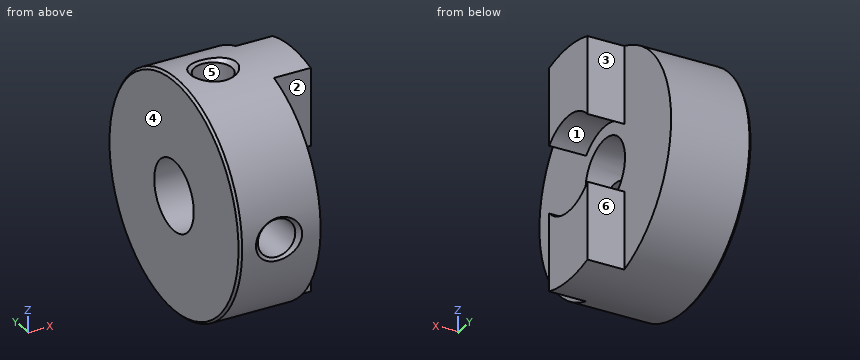
from build123d import *

# Parameters (mm, degrees)
SKETCH2_W          = 3.2
SKETCH2_H          = 4.1
SKETCH3_W          = 22
SKETCH3_H          = 21
SKETCH3_W_2        = 20
SKETCH3_H_2        = 5.8
CUT_EXTRUDE1_DEPTH = 3.2


with BuildPart() as part:
    # Sketch1 → Revolve1 (revolve)
    with BuildSketch(Plane.XY):
        Polygon((0, 9.8), (0, 3), (10.2, 3), (10.2, 10), (0.2, 10), align=None)
    revolve(axis=Axis((10.2, 0, 0), (-1, 0, 0)))

    # Sketch2 → Cut-Revolve1 (revolve, cut)
    with BuildSketch(Plane.XY):
        with Locations((8.6, 2.05)):
            Rectangle(SKETCH2_W, SKETCH2_H)
    revolve(axis=Axis((10.2, 0, 0), (-1, 0, 0)), mode=Mode.SUBTRACT)

    # Sketch3 → Cut-Extrude1 (cut)
    with BuildSketch(Plane(origin=(10.2, 0, 0), x_dir=(0, 0, -1), z_dir=(1, 0, 0))):
        Rectangle(SKETCH3_W, SKETCH3_H)
        Rectangle(SKETCH3_W_2, SKETCH3_H_2, mode=Mode.SUBTRACT)
    extrude(amount=-CUT_EXTRUDE1_DEPTH, mode=Mode.SUBTRACT)

    # Sketch4 → Cut-Revolve2 (revolve, cut)
    with BuildSketch(Plane(origin=(3.4, 0, 0), x_dir=(0, 0, -1), z_dir=(1, 0, 0))):
        Polygon((-10, 0), (-10, 2), (-9.621, 1.621), (0, 1.621), (0, 0), align=None)
    revolve(axis=Axis((3.4, 0, 0), (0, 0, 1)), mode=Mode.SUBTRACT)

    # Sketch5 → Cut-Revolve3 (revolve, cut)
    with BuildSketch(Plane(origin=(3.4, 0, 0), x_dir=(0, 0, -1), z_dir=(1, 0, 0))):
        Polygon((0, -10), (-2, -10), (-1.621, -9.621), (-1.621, 0), (0, 0), align=None)
    revolve(axis=Axis((3.4, 0, 0), (0, -1, 0)), mode=Mode.SUBTRACT)


solid = part.part
Source: CAD feature listing. Evaluate the final solid. Frame: model axes, mm. Face numbers are marked on the shaded views. A direction names the side the tool comes from. Coordinates: 2 decimals unless noted, no trailing zeros. Write each loop counter-clockwise with the first axis right and the second up, starting at its lowest first coordinate (ties: lowest second). Pieces come first, ordered by that corner, then holes. Notation, with made-up numbers: M 48.25,64 L 99.25,64 A11 cw 99.25,78 Z; hole C -15,87 d4. An arc over 180 degrees is marked long. Use a Markdown table: item, result.
1) Ray query, L1, parallel to Y at x = 2, z = 0; L2, parallel to X at y = 6.25, z = -1.25; L3, parallel to Z at x = 1.75, y = 2.75. Return the intervals inside material, ascending.
Conclusion:
| item | result |
|---|---|
| L1 | y = 3 to 10 |
| L2 | x = 0 to 7 |
| L3 | z = -9.61 to -1.2, 1.2 to 9.61 |
2) Mould query, pull axis Y, two halves, no side actions, for the marked faces 4, 5 and 6. Classes: pulls with the +Y half, pulls with the -Y half, needs draft (parallel to the pull), parting line crosses it, or undercut.
Conclusion:
| item | result |
|---|---|
| face 4 | needs draft |
| face 5 | undercut |
| face 6 | pulls with the +Y half |
3) First-contact query: pin 1 Ø10 at (y, z) = (5, 6) entering from -X; pin 2 Ø6 at (x, z) = (2.5, 3) entering from -Y; pin 3 Ø1.6 at (x, z) = (8.5, -5.5) entering from +Y; pin 4 Ø6 at (x, y) = (6, -4) entering from -Z. Flat tips, straight axial feed; report the tip coordinate or a pass-through.
Conclusion:
| item | result |
|---|---|
| pin 1 | stops at x = 0 |
| pin 2 | stops at y = -10 |
| pin 3 | stops at y = 2.9 |
| pin 4 | stops at z = -9.95 |
4) Section C-C, the plane x = 8.25. Output: boundary loops of the cut face in (y, z), then the cut area to 3 significant figures.
Conclusion:
| item | result |
|---|---|
| outline | M -2.9,-9.57 A10 ccw 2.9,-9.57 L 2.9,-2.9 A4.1 cw -2.9,-2.9 Z; M -2.9,2.9 A4.1 cw 2.9,2.9 L 2.9,9.57 A10 ccw -2.9,9.57 Z |
| area | 71.1 mm^2 |
5) Section A-A, the plane y = 0. Output: boundary loops of the cut face in (x, z).
Conclusion:
| item | result |
|---|---|
| outline | M 0,-9.8 L 0.2,-10 L 10.2,-10 L 10.2,-4.1 L 7,-4.1 L 7,-3 L 0,-3 Z; M 0,3 L 1.78,3 L 1.78,9.62 L 1.4,10 L 0.2,10 L 0,9.8 Z; M 5.02,3 L 7,3 L 7,4.1 L 10.2,4.1 L 10.2,10 L 5.4,10 L 5.02,9.62 Z |
6) Section B-B, the plane z = 0. Output: boundary loops of the cut face in (x, y), then the cut area to 3 significant figures.
Conclusion:
| item | result |
|---|---|
| outline | M 0,-9.8 L 0.2,-10 L 1.4,-10 L 1.78,-9.62 L 1.78,-3 L 0,-3 Z; M 0,3 L 7,3 L 7,10 L 0.2,10 L 0,9.8 Z; M 5.02,-9.62 L 5.4,-10 L 7,-10 L 7,-3 L 5.02,-3 Z |
| area | 75.1 mm^2 |
7) Section D-D, the plane x = 3.4. Output: boundary loops of the cut face in (y, z), then the cut area to 3 significant figures.
Conclusion:
| item | result |
|---|---|
| outline | M -9.83,-1.83 A10 ccw long 1.83,9.83 L 1.62,9.62 L 1.62,2.52 A3 cw long -2.52,-1.62 L -9.62,-1.62 Z; M -9.83,1.83 L -9.62,1.62 L -2.52,1.62 A3 cw -1.62,2.52 L -1.62,9.62 L -1.83,9.83 A10 ccw Z |
| area | 240 mm^2 |
8) Reachability of the marked faces 1, 2 and 3 from +Z, -Z, +X, -X, +Y, -Y: full face, straight path, thin tool, end or side. Return the list, or none.
Conclusion:
| item | result |
|---|---|
| face 1 | +X |
| face 2 | +Z, -Z, +X, -Y |
| face 3 | +Z, -Z, +X, +Y |
